```python
from build123d import *

# Parameters (mm, degrees)
SKETCH1_R           = 6
SKETCH1_R_2         = 1.5
SKETCH1_R_3         = 1.25
BOSS_EXTRUDE1_DEPTH = 3.75
SKETCH2_R           = 7
CUT_EXTRUDE1_DEPTH  = 2
CUT_EXTRUDE2_DEPTH  = 1
SKETCH4_R           = 1.5
CUT_EXTRUDE3_DEPTH  = 10


with BuildPart() as part:
    # Sketch1 → Boss-Extrude1 (new body)
    with BuildSketch(Plane.XY):
        with BuildLine():
            Line((-14.999999511, 12.999998728), (-14.999999511, -12.999999576))
            Line((-14.999999511, -12.999999576), (15.000000489, -12.999999576))
            Line((15.000000489, -12.999999576), (15.000000489, 13.000000424))
            ThreePointArc((15.000000489, 13.000000424), (-3.59e-07, 28), (-14.999999511, 12.999998728))
        make_face()
        with Locations((4.89e-07, 13)):
            Circle(SKETCH1_R, mode=Mode.SUBTRACT)
        with Locations((-9.499999511, 13)):
            Circle(SKETCH1_R_2, mode=Mode.SUBTRACT)
        with Locations((9.500000489, 13)):
            Circle(SKETCH1_R_2, mode=Mode.SUBTRACT)
        with Locations((-7.5, -3)):
            Circle(SKETCH1_R_3, mode=Mode.SUBTRACT)
        with Locations((7.5, -3)):
            Circle(SKETCH1_R_3, mode=Mode.SUBTRACT)
        with Locations((10.000000489, 2)):
            Circle(SKETCH1_R_3, mode=Mode.SUBTRACT)
        with Locations((-9.999999511, 2)):
            Circle(SKETCH1_R_3, mode=Mode.SUBTRACT)
        with Locations((0, 2)):
            Circle(SKETCH1_R_3, mode=Mode.SUBTRACT)
        with Locations((0, -4.4)):
            Circle(SKETCH1_R_3, mode=Mode.SUBTRACT)
    extrude(amount=BOSS_EXTRUDE1_DEPTH)

    # Sketch2 → Cut-Extrude1 (cut)
    with BuildSketch(Plane.XY.offset(3.75)):
        with Locations((4.89e-07, 13)):
            Circle(SKETCH2_R)
    extrude(amount=-CUT_EXTRUDE1_DEPTH, mode=Mode.SUBTRACT)

    # Sketch3 → Cut-Extrude2 (cut)
    with BuildSketch(Plane.XY):
        with BuildLine():
            Line((15.000000489, -12.999999576), (15.000000489, 13.000000424))
            ThreePointArc((15.000000489, 13.000000424), (-3.59e-07, 28), (-14.999999511, 12.999998728))
            Line((-14.999999511, 12.999998728), (-14.999999511, -12.999999576))
            Line((-14.999999511, -12.999999576), (15.000000489, -12.999999576))
        make_face()
        with BuildLine():
            Line((-13.499999511, 12.999998855), (-13.499999511, -11.499999576))
            Line((-13.499999511, -11.499999576), (13.500000489, -11.499999576))
            Line((13.500000489, -11.499999576), (13.500000489, 13.000000382))
            ThreePointArc((13.500000489, 13.000000382), (-2.74e-07, 26.5), (-13.499999511, 12.999998855))
        make_face(mode=Mode.SUBTRACT)
    extrude(amount=CUT_EXTRUDE2_DEPTH, mode=Mode.SUBTRACT)

    # Sketch4 → Cut-Extrude3 (cut)
    with BuildSketch(Plane.XY.offset(3.75)):
        with Locations((-9.526278952, 18.5)):
            Circle(SKETCH4_R)
        with Locations((9.526280345, 18.499999283)):
            Circle(SKETCH4_R)
    extrude(amount=-CUT_EXTRUDE3_DEPTH, mode=Mode.SUBTRACT)


solid = part.part
```
Check sheet for the modelled part. Datum: model origin and axes. Units: mm. A direction names the side the tool comes from. Give positions to 0.01 mm unless a question says otherwise; leave off trailing zeros. Write each loop counter-clockwise with the first axis right and the second up, starting at its lowest first coordinate (ties: lowest second). Pieces come first, ordered by that corner, then holes. Notation, with made-up numbers: (4.25, 63) - (48.25, 63) arc R23 ccw to (48.25, 92) - close; hole circle Ø5 at (81.25, -37.5). An arc over 180 degrees is marked (long way). Answer as a JSON object with one key per item and string values. Group by question number.
1) Sectioned sample at B-B (x = 10). Record the cut outline in (y, z).
2) Sectioned sample at D-D (y = -8.5). Record the cut outline in (x, z).
3) Release check for a two-part mould opening along X. For faces 4 (the face through (-8.421, -2.155, 1.849)), 5 (the face through (13.5, 0.6, 0.5)), 6 (the face through (0.297, 26.497, 0.493)) record: pulls with the +X half, pulls with the -X half, needs draft (parallel to the pull), parting line crosses it, or undercut.
4) Sectioned sample at A-A (y = 2). Record the cut outline in (x, z).
5) Depth check by flat-ended pin: P1, Ø12, axis at x = -7, y = 22.5, coming from the -Z side; P2, Ø0.5, axis at y = -5, z = 0.5, coming from the -X side; P3, Ø0.5, axis at x = 5.5, z = 0.5, coming from the -Y side. Enter the tip coordinate at first touch or a pass-through.
6) Access from +Z, -Z, +X, -X, +Y, -Y to the whole of each face (thin tool, end or side, straight path). Record for faces 1 (the face through (-1.517, 6.166, 2.764)), 2 (the face through (-13.5, 0.9, 0.5)), 3 (the face through (-0.2, -11.5, 0.5)).
7) Thickness scan on probe 1 along Y at (x, z) = (0, 1.3); probe 2 along Y at (x, z) = (9.5, 2.15); probe 3 along Y at (x, z) = (-3, 3.35). Record the ranges inside material, lowest first. Write a range as from..to.
8) Sectioned sample at C-C (z = 2.8). Give the number of separate pieces and of enclosed holes in the cut face, then the cut area to 3 significant figures.
Geometry results:
{
 "1": {"outline": "(-13, 1) - (-11.5, 1) - (-11.5, 0) - (0.75, 0) - (0.75, 3.75) - (-13, 3.75) - close; (3.25, 0) - (11.59, 0) - (11.59, 3.75) - (3.25, 3.75) - close; (14.41, 0) - (17.08, 0) - (17.08, 3.75) - (14.41, 3.75) - close; (19.92, 0) - (22.07, 0) - (22.07, 1) - (24.18, 1) - (24.18, 3.75) - (19.92, 3.75) - close"},
 "2": {"outline": "(-15, 1) - (-13.5, 1) - (-13.5, 0) - (13.5, 0) - (13.5, 1) - (15, 1) - (15, 3.75) - (-15, 3.75) - close"},
 "3": {"face 4": "undercut", "face 5": "pulls with the +X half", "face 6": "parting line crosses it"},
 "4": {"outline": "(-15, 1) - (-13.5, 1) - (-13.5, 0) - (-11.25, 0) - (-11.25, 3.75) - (-15, 3.75) - close; (-8.75, 0) - (-1.25, 0) - (-1.25, 3.75) - (-8.75, 3.75) - close; (1.25, 0) - (8.75, 0) - (8.75, 3.75) - (1.25, 3.75) - close; (11.25, 0) - (13.5, 0) - (13.5, 1) - (15, 1) - (15, 3.75) - (11.25, 3.75) - close"},
 "5": {"P1": "stops at z = 0", "P2": "stops at x = -13.5", "P3": "stops at y = -11.5"},
 "6": {"face 1": "+Z", "face 2": "-Z, -X, +Y, -Y", "face 3": "-Z, +X, -X, -Y"},
 "7": {"probe 1": "y = -13..-5.65, -3.15..0.75, 3.25..7, 19..28", "probe 2": "y = -13..0.85, 3.15..11.5, 14.5..17, 20..24.61", "probe 3": "y = -13..6.68, 19.32..27.7"},
 "8": {"separate pieces": "1", "enclosed holes": "11", "area": "922 mm^2"}
}
